from build123d import *

# Parameters (mm, degrees)
BOSS_EXTRUDE1_DEPTH = 3.175
SKETCH2_R           = 3.175
CUT_EXTRUDE1_DEPTH  = 3.175
LPATTERN1_COUNT     = 3
LPATTERN1_PITCH     = 25.4
LPATTERN2_COUNT     = 2
LPATTERN2_PITCH     = 25.4


with BuildPart() as part:
    # Sketch1 → Boss-Extrude1 (new body)
    with BuildSketch(Plane(origin=(0, 0, 0), x_dir=(1, 0, 0), z_dir=(0, 1, 0))):
        Polygon((0, 0), (0, 76.2), (25.4, 76.2), (25.4, 25.429586946), (50.8, 25.429586946), (50.8, 0), align=None)
    extrude(amount=BOSS_EXTRUDE1_DEPTH)

    # Sketch2 → Cut-Extrude1 (cut)
    with BuildSketch(Plane(origin=(0, 3.175, 0), x_dir=(1, 0, 0), z_dir=(0, 1, 0))):
        with Locations(Location((12.7, 12.7, 0), (0, 0, 270))):
            Circle(SKETCH2_R)
    cut_extrude1 = extrude(amount=-CUT_EXTRUDE1_DEPTH, mode=Mode.SUBTRACT)

    # LPattern1: Cut-Extrude1 ×3
    with Locations(*[(0, 0, -i * LPATTERN1_PITCH) for i in range(1, LPATTERN1_COUNT)]):
        add(cut_extrude1, mode=Mode.SUBTRACT)

    # LPattern2: Cut-Extrude1 ×2
    with Locations(*[(i * LPATTERN2_PITCH, 0, 0) for i in range(1, LPATTERN2_COUNT)]):
        add(cut_extrude1, mode=Mode.SUBTRACT)


solid = part.part
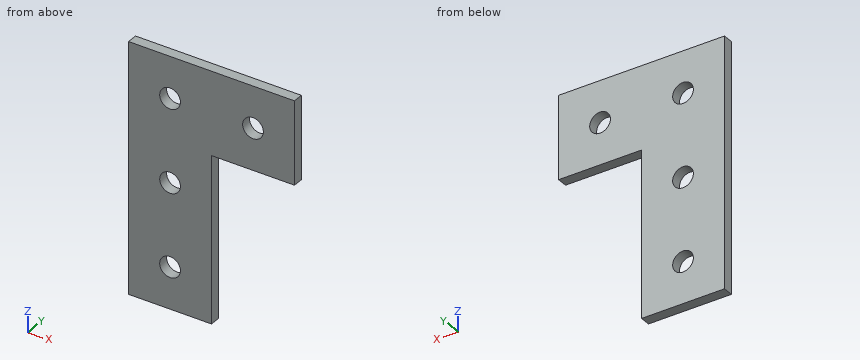
Input: part model. Units: mm. Frame: model coordinates. Give positions to 0.01 mm unless a question says otherwise; leave off trailing zeros. Order: outer loops, then holes, each group sorted by start corner. A loop starts at its lowest first (then second) coordinate and runs counter-clockwise, first axis right, second up. Notation, with made-up numbers: M 49,-21.5 L 69,-21.5 A12 ccw 69,-14.5 Z; hole C -20,86 d10. An arc over 180 degrees is marked long. Answer as a JSON object with one key per item and string values.
1. Cut plane B-B, the plane z = -63.5. Output: boundary loops of the cut face in (x, y) (3 decimals), and give its area (3 significant figures).
Result sheet:
{"outline": "M 0,0 L 9.525,0 L 9.525,3.175 L 0,3.175 Z; M 15.875,0 L 25.4,0 L 25.4,3.175 L 15.875,3.175 Z", "area": "60.5 mm²"}
2. Cut plane D-D, the plane x = 12.7. Output: boundary loops of the cut face in (y, z) (3 decimals), and give its area (3 significant figures).
Result sheet:
{"outline": "M 0,-76.2 L 3.175,-76.2 L 3.175,-66.675 L 0,-66.675 Z; M 0,-60.325 L 3.175,-60.325 L 3.175,-41.275 L 0,-41.275 Z; M 0,-34.925 L 3.175,-34.925 L 3.175,-15.875 L 0,-15.875 Z; M 0,-9.525 L 3.175,-9.525 L 3.175,0 L 0,0 Z", "area": "181 mm²"}
3. Cut plane C-C, the plane y = 2.65. Output: boundary loops of the cut face in (x, z) (3 decimals), and give its area (3 significant figures).
Result sheet:
{"outline": "M 0,-76.2 L 25.4,-76.2 L 25.4,-25.43 L 50.8,-25.43 L 50.8,0 L 0,0 Z; hole C 12.7,-63.5 d6.35; hole C 12.7,-38.1 d6.35; hole C 12.7,-12.7 d6.35; hole C 38.1,-12.7 d6.35", "area": "2,450 mm²"}
4. First-contact query: P1, Ø12, axis at x = 45.5, z = -36, coming from the +Y side; P2, Ø1.6, axis at x = 42, y = 2, coming from the -Z side; P3, Ø1.5, axis at y = 2.5, z = -25.5, coming from the +X side. Flat tips, straight axial feed; report the tip coordinate or a pass-through.
Result sheet:
{"P1": "through", "P2": "z = -25.43", "P3": "x = 50.8"}
5. Cut plane A-A, the plane z = -12.7. Output: boundary loops of the cut face in (x, y) (3 decimals).
Result sheet:
{"outline": "M 0,0 L 9.525,0 L 9.525,3.175 L 0,3.175 Z; M 15.875,0 L 34.925,0 L 34.925,3.175 L 15.875,3.175 Z; M 41.275,0 L 50.8,0 L 50.8,3.175 L 41.275,3.175 Z"}
6. Ray query, line 1 (X direction, y = 2.25, z = -12.7) (3 decimals); line 2 (X direction, y = 1.85, z = -38.1) (3 decimals); line 3 (X direction, y = 2.75, z = -27). Return the intervals inside material, ascending. Write a range as [from, to].
Result sheet:
{"line 1": "[0, 9.525], [15.875, 34.925], [41.275, 50.8]", "line 2": "[0, 9.525], [15.875, 25.4]", "line 3": "[0, 25.4]"}
